from build123d import *

# Parameters (mm, degrees)
SKETCH1_R           = 14
BOSS_EXTRUDE1_DEPTH = 4
SKETCH2_R           = 2.94
BOSS_EXTRUDE2_DEPTH = 7
SKETCH4_R           = 11
CUT_EXTRUDE1_DEPTH  = 1
FILLET1_R           = 0.5


with BuildPart() as part:
    # Sketch1 → Boss-Extrude1 (new body)
    with BuildSketch(Plane.XY):
        Circle(SKETCH1_R)
    extrude(amount=BOSS_EXTRUDE1_DEPTH)

    # Sketch2 → Boss-Extrude2 (add)
    with BuildSketch(Plane.XY.offset(4)):
        Circle(SKETCH2_R)
    extrude(amount=BOSS_EXTRUDE2_DEPTH)

    # Sketch4 → Cut-Extrude1 (cut)
    with BuildSketch(Plane(origin=(0, 0, 0), x_dir=(-1, 0, 0), z_dir=(0, 0, -1))):
        Circle(SKETCH4_R)
    extrude(amount=-CUT_EXTRUDE1_DEPTH, mode=Mode.SUBTRACT)

    # Fillet1
    fillet1_edges = [part.edges().sort_by_distance(p)[0] for p in [
        (11, 0, 1),
        (11, 0, 0),
    ]]
    fillet(fillet1_edges, radius=FILLET1_R - 0.0001)  # a hair under: the kernel refuses the full size


solid = part.part
Could you check a few things on this model? Use its own coordinates, in mm. Round coordinates to 2 decimals unless told otherwise and drop trailing zeros. Order: outer loops, then holes, each group sorted by start corner. A loop starts at its lowest first (then second) coordinate and runs counter-clockwise, first axis right, second up.
Q1. Thinking about a two-plate mould opening in X: for faces 1 (the face through (2.8, 0.9, 7.5)), 2 (the face through (2, 11.5, 0)), 3 (the face through (0, 0, 1)), which applies, released by +X, released by -X, zero draft, split by the parting line, or undercut?
Geometry says:
face 1: split by the parting line
face 2: zero draft
face 3: undercut
Q2. Imagine slicing it at C-C, the plane z = 4.75. List the corners of the cut face in (x, y) for me.
Geometry says:
outline: circle Ø5.88 at (0, 0)
Q3. I'm going to push flat-ended pins straight in: P1, Ø3, axis at x = -3.5, z = 6.5, coming from the -Y side; P2, Ø6, axis at x = -5.5, y = 3, coming from the +Z side; P3, Ø1, axis at x = 8, y = -1, coming from the -Z side. Where does each tip first touch, or does it pass through?
Geometry says:
P1: stops at y = -2.15
P2: stops at z = 4
P3: stops at z = 1
Q4. Please list where these lines run through material, in increasing order: probe 1 along Y at (x, z) = (0, 0.55); probe 2 along Z at (x, y) = (10.5, 7.5); probe 3 along Z at (x, y) = (-9.5, 3.75).
Geometry says:
probe 1: y = -14 to -11, 11 to 14
probe 2: z = 0 to 4
probe 3: z = 1 to 4
